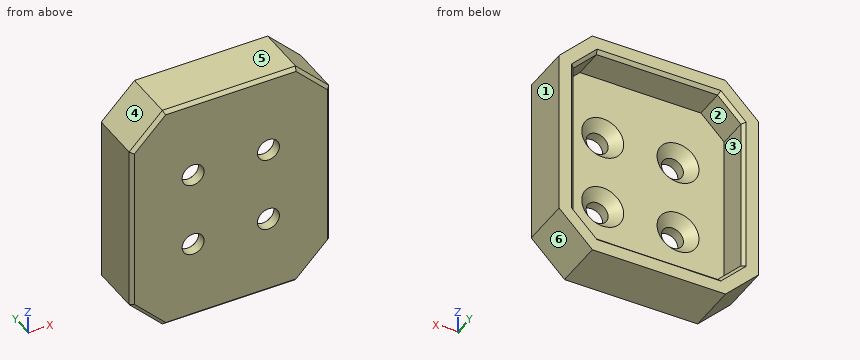
from build123d import *

# Parameters (mm, degrees)
SKETCH1_W                                      = 30
SKETCH1_H                                      = 35
BOSS_EXTRUDE1_DEPTH                            = 3
SKETCH2_W                                      = 30
SKETCH2_H                                      = 35
BOSS_EXTRUDE2_DEPTH                            = 5
CHAMFER1_SIZE                                  = 5
CSK_FOR_M3_FLAT_HEAD_MACHINE_SCREW1_AT_2_COUNT = 2
CSK_FOR_M3_FLAT_HEAD_MACHINE_SCREW1_AT_2_PITCH = 11.313708499
CSK_FOR_M3_FLAT_HEAD_MACHINE_SCREW1_AT_3_COUNT = 2
CSK_FOR_M3_FLAT_HEAD_MACHINE_SCREW1_AT_3_PITCH = 16
CSK_FOR_M3_FLAT_HEAD_MACHINE_SCREW1_AT_4_COUNT = 2
CSK_FOR_M3_FLAT_HEAD_MACHINE_SCREW1_AT_4_PITCH = 11.313708499
CHAMFER2_SIZE                                  = 0.5
CHAMFER3_SIZE                                  = 0.5


with BuildPart() as part:
    # Sketch1 → Boss-Extrude1 (new body)
    with BuildSketch(Plane(origin=(0, 0, 0), x_dir=(1, 0, 0), z_dir=(0, 1, 0))):
        Rectangle(SKETCH1_W, SKETCH1_H)
    extrude(amount=BOSS_EXTRUDE1_DEPTH)

    # Sketch2 → Boss-Extrude2 (add)
    with BuildSketch(Plane(origin=(0, 3, 0), x_dir=(1, 0, 0), z_dir=(0, 1, 0))):
        Rectangle(SKETCH2_W, SKETCH2_H)
        Polygon((12.6, -11.6), (12.6, 11.6), (9.1, 15.1), (-9.1, 15.1), (-12.6, 11.6), (-12.6, -11.6), (-9.1, -15.1), (9.1, -15.1), align=None, mode=Mode.SUBTRACT)
    extrude(amount=BOSS_EXTRUDE2_DEPTH)

    # Chamfer1
    chamfer1_edges = [part.edges().sort_by_distance(p)[0] for p in [
        (15, 4, 17.5),
        (-15, 4, 17.5),
        (-15, 4, -17.5),
        (15, 4, -17.5),
    ]]
    chamfer(chamfer1_edges, length=CHAMFER1_SIZE)

    # Sketch6 → CSK for M3 Flat Head Machine Screw1 (revolve, cut)
    with BuildSketch(Plane(origin=(-5.656854249, 3, -5.656854249), x_dir=(0, 0, 1), z_dir=(1, 0, 0))):
        Polygon((0, 0), (0, 3), (1.65, 3), (1.65, 1.5), (3.15, 0), align=None)
    csk_for_m3_flat_head_machine_screw1 = revolve(axis=Axis((-5.656854249, 9.35, -5.656854249), (0, -1, 0)), mode=Mode.SUBTRACT)

    # CSK for M3 Flat Head Machine Screw1 at 2: CSK for M3 Flat Head Machine Screw1 ×2
    with Locations(*[(i * CSK_FOR_M3_FLAT_HEAD_MACHINE_SCREW1_AT_2_PITCH, 0, 0) for i in range(1, CSK_FOR_M3_FLAT_HEAD_MACHINE_SCREW1_AT_2_COUNT)]):
        add(csk_for_m3_flat_head_machine_screw1, mode=Mode.SUBTRACT)

    # CSK for M3 Flat Head Machine Screw1 at 3: CSK for M3 Flat Head Machine Screw1 ×2
    with Locations(*[Vector(0.707106781, 0, 0.707106781) * (i * CSK_FOR_M3_FLAT_HEAD_MACHINE_SCREW1_AT_3_PITCH) for i in range(1, CSK_FOR_M3_FLAT_HEAD_MACHINE_SCREW1_AT_3_COUNT)]):
        add(csk_for_m3_flat_head_machine_screw1, mode=Mode.SUBTRACT)

    # CSK for M3 Flat Head Machine Screw1 at 4: CSK for M3 Flat Head Machine Screw1 ×2
    with Locations(*[(0, 0, i * CSK_FOR_M3_FLAT_HEAD_MACHINE_SCREW1_AT_4_PITCH) for i in range(1, CSK_FOR_M3_FLAT_HEAD_MACHINE_SCREW1_AT_4_COUNT)]):
        add(csk_for_m3_flat_head_machine_screw1, mode=Mode.SUBTRACT)

    # Chamfer2
    chamfer2_edges = [part.edges().sort_by_distance(p)[0] for p in [
        (-10.85, 8, -13.35),
        (-12.6, 8, 0),
        (-10.85, 8, 13.35),
        (0, 8, 15.1),
        (10.85, 8, 13.35),
        (12.6, 8, 0),
        (10.85, 8, -13.35),
        (0, 8, -15.1),
    ]]
    chamfer(chamfer2_edges, length=CHAMFER2_SIZE)

    # Chamfer3
    chamfer3_edges = [part.edges().sort_by_distance(p)[0] for p in [
        (15, 0, 0),
        (0, 0, 17.5),
        (-15, 0, 0),
        (0, 0, -17.5),
        (-12.5, 0, -15),
        (12.5, 0, -15),
        (-12.5, 0, 15),
        (12.5, 0, 15),
    ]]
    chamfer(chamfer3_edges, length=CHAMFER3_SIZE)


solid = part.part
For this review, take the finished solid that the model builds, in its own axes (mm). Face numbers are marked on the shaded views. A direction names the side the tool comes from. Coordinates: 2 decimals unless noted, no trailing zeros. Order: outer loops, then holes, each group sorted by start corner. A loop starts at its lowest first (then second) coordinate and runs counter-clockwise, first axis right, second up. Notation, with made-up numbers: (-36.5, 61.25) - (20.5, 61.25) arc R7 ccw to (20.5, 65.25) - close; hole circle Ø6 at (-32.75, 59.25). An arc over 180 degrees is marked (long way). Use one line per item in the form item = value.
Q1. Consider section B-B (z = 10.5). Give the boundary of the cut face in (x, y), then the cut area to 4 significant figures.
Checked values:
outline = (-15, 0.5) - (-14.5, 0) - (14.5, 0) - (15, 0.5) - (15, 8) - (13.1, 8) - (12.6, 7.5) - (12.6, 3) - (-12.6, 3) - (-12.6, 7.5) - (-13.1, 8) - (-15, 8) - close
area = 113.5 mm2
Q2. For probe 1 along X at (y, z) = (4.5, 0.5); probe 2 along Z at (x, y) = (6, 5.5); probe 3 along X at (y, z) = (2.75, 6), list the stretches that pass through material, from the lowest coordinate up. Write a range as from..to.
Checked values:
probe_1 = -15..-12.6, 12.6..15
probe_2 = -17.5..-15.1, 15.1..17.5
probe_3 = -15..-8.54, -2.78..2.78, 8.54..15
Q3. Consider section A-A (x = 2). Give the boundary of the cut face in (y, z).
Checked values:
outline = (0, -17) - (0.5, -17.5) - (8, -17.5) - (8, -15.6) - (7.5, -15.1) - (3, -15.1) - (3, 15.1) - (7.5, 15.1) - (8, 15.6) - (8, 17.5) - (0.5, 17.5) - (0, 17) - close
Q4. Draft analysis for pull direction X (two halves, no side actions). For the marked faces 3, 4, 5 and 6, state which applies: +X half, -X half, draft (parallel to the pull), parting line (faces both ways), or undercut.
Checked values:
face_3 = undercut
face_4 = -X half
face_5 = draft
face_6 = +X half
Q5. For the marked faces 1 and 2, list the 3-axis set-ups (+Z, -Z, +X, -X, +Y, -Y) from which the entire face can be reached by the end or side of a thin tool; tool diameter is ignored.
Checked values:
face_1 = +Z, -Z, +X, +Y, -Y
face_2 = +Y
Q6. For P1, Ø4, axis at x = -5.66, z = 5.66, coming from the +Y side; P2, Ø5.5, axis at x = 5.66, z = 5.66, coming from the +Y side, all flat-tipped, find the tip position at first contact; note any pin that passes through.
Checked values:
P1 = 1.85
P2 = 2.6
Q7. Consider section D-D (y = 1). Give the boundary of the cut face in (x, z), then the cut area to 3 significant figures.
Checked values:
outline = (-15, -12.5) - (-10, -17.5) - (10, -17.5) - (15, -12.5) - (15, 12.5) - (10, 17.5) - (-10, 17.5) - (-15, 12.5) - close; hole circle Ø3.3 at (-5.66, -5.66); hole circle Ø3.3 at (-5.66, 5.66); hole circle Ø3.3 at (5.66, -5.66); hole circle Ø3.3 at (5.66, 5.66)
area = 966 mm2
Q8. Consider section C-C (y = 3.75). Give the boundary of the cut face in (x, z).
Checked values:
outline = (-15, -12.5) - (-10, -17.5) - (10, -17.5) - (15, -12.5) - (15, 12.5) - (10, 17.5) - (-10, 17.5) - (-15, 12.5) - close; hole (-12.6, -11.6) - (-9.1, -15.1) - (9.1, -15.1) - (12.6, -11.6) - (12.6, 11.6) - (9.1, 15.1) - (-9.1, 15.1) - (-12.6, 11.6) - close
